Autodesk Inventor part; units mm, degrees
ref_plane "YZ Plane" through (0, 0, 0) normal (1, 0, 0) x (0, 1, 0)
ref_plane "XZ Plane" through (0, 0, 0) normal (0, 1, 0) x (-1, 0, 0)
ref_plane "XY Plane" through (0, 0, 0) normal (0, 0, 1) x (1, 0, 0)
sketch "Sketch1" plane through (0, 0, 0) normal (0, 1, 0) x (-1, 0, 0)
  line L0 (25, 15) -> (-25, 15)
  line L1 (-25, 15) -> (-25, -15)
  line L2 (-25, -15) -> (25, -15)
  line L3 (25, -15) -> (25, 15)
  line L4 (25, 15) -> (-25, -15) construction
  line L5 (-25, 15) -> (25, -15) construction
  point P0 (0, 0)
  dimension "d0" = 50
  dimension "d1" = 30
extrude "Extrusion1" add sketch "Sketch1" along normal mid plane 230
fillet "Fillet1" radius 3 4 edges at (25, 0, 15) (25, 0, -15) (-25, 0, 15) (-25, 0, -15)
shell "Shell1" thickness 1.2 removed faces 2 at (-7.3333, 115, -5) at (-7.3333, -115, -5)
properties part number "Perfil 30x501"
Input: part model. Units: mm. Frame: model coordinates. A direction names the side the tool comes from. Round coordinates to 2 decimals unless told otherwise and drop trailing zeros. Loops run counter-clockwise (first coordinate to the right, second up) from the corner with the lowest first, then second, coordinate; pieces in that order, holes last. Notation, with made-up numbers: (77.25, 3.5) -> (96.25, 3.5) arc R17 cw to (96.25, 7.5) -> close; hole circle Ø8 at (73, -25.5). An arc over 180 degrees is marked (long way). Answer as a JSON object with one key per item and string values. Group by question number.
1) Ray query, L1, parallel to X at y = -25.5, z = -3.5; L2, parallel to Z at x = 8.5, y = 32; L3, parallel to X at y = -103, z = 13.5. Return the intervals inside material, ascending.
2) Draft query along X for faces 1 (the flat face through (0.1, -115, 14.5)), 2 (the flat face through (0, -2, 13.8)), 3 (the flat face through (25, -2, 0)). Return one class per face: +X half, -X half, draft (parallel to the pull), parting line (faces both ways), or undercut.
3) Section query B-B on x = -4.5. Output: boundary loops of the cut face in (y, z).
4) Section query A-A on z = 2.5. Output: boundary loops of the cut face in (x, y), plus the area to 3 significant figures.
5) Pin query (flat end, axial travel): pin 1 (6 mm diameter, centred on x = 19, z = 6.5, fed in from +Y). Return the tip coordinate at first contact, or that it passes through.
6) Reachability of faces 4 (the flat face through (23.8, -2, 0)), 5 (the flat face through (-25, -2, 0)) from +Z, -Z, +X, -X, +Y, -Y: full face, straight path, thin tool, end or side. Return the list, or none.
7) Section query C-C on y = -70. Output: boundary loops of the cut face in (x, z).
Reply:
{
 "1": {"L1": "x = -25 to -23.8, 23.8 to 25", "L2": "z = -15 to -13.8, 13.8 to 15", "L3": "x = -24.6 to -22.99, 22.99 to 24.6"},
 "2": {"face 1": "draft", "face 2": "undercut", "face 3": "+X half"},
 "3": {"outline": "(-115, -15) -> (115, -15) -> (115, -13.8) -> (-115, -13.8) -> close; (-115, 13.8) -> (115, 13.8) -> (115, 15) -> (-115, 15) -> close"},
 "4": {"outline": "(-25, -115) -> (-23.8, -115) -> (-23.8, 115) -> (-25, 115) -> close; (23.8, -115) -> (25, -115) -> (25, 115) -> (23.8, 115) -> close", "area": "552 mm2"},
 "5": {"pin 1": "passes through"},
 "6": {"face 4": "+Y, -Y", "face 5": "+Z, -Z, -X, +Y, -Y"},
 "7": {"outline": "(-25, -12) arc R3 ccw to (-22, -15) -> (22, -15) arc R3 ccw to (25, -12) -> (25, 12) arc R3 ccw to (22, 15) -> (-22, 15) arc R3 ccw to (-25, 12) -> close; hole (-23.8, -12) arc R1.8 ccw to (-22, -13.8) -> (22, -13.8) arc R1.8 ccw to (23.8, -12) -> (23.8, 12) arc R1.8 ccw to (22, 13.8) -> (-22, 13.8) arc R1.8 ccw to (-23.8, 12) -> close"}
}
